```python
from build123d import *

# Parameters (mm, degrees)
BOSS_EXTRUDE1_DEPTH = 14.5
SKETCH3_R           = 4.1
CUT_EXTRUDE1_DEPTH  = 4
BOSS_EXTRUDE2_START = 2
SKETCH5_R           = 14.5
SKETCH5_R_2         = 4.1
BOSS_EXTRUDE2_DEPTH = 2
SKETCH6_R           = 1.55
CUT_EXTRUDE3_DEPTH  = 3
SKETCH7_R           = 10.5
CUT_EXTRUDE4_DEPTH  = 3
FILLET1_R           = 14.5
CUT_EXTRUDE5_DEPTH  = 3
SKETCH9_R           = 1.55
CUT_EXTRUDE6_DEPTH  = 3
SKETCH10_R          = 3
CUT_EXTRUDE7_DEPTH  = 2
SKETCH13_W          = 33
SKETCH13_H          = 3
CUT_EXTRUDE8_DEPTH  = 29


with BuildPart() as part:
    # Sketch2 → Boss-Extrude1 (new, symmetric)
    with BuildSketch(Plane.XY):
        Polygon((-63.7, 18.3), (-4.658041958, 18.3), (10, 3), (43, 3), (43, 0), (0, 0), (-13.7, 14.3), (-63.7, 14.3), align=None)
    extrude(amount=BOSS_EXTRUDE1_DEPTH, both=True)

    # Sketch3 → Cut-Extrude1 (cut)
    with BuildSketch(Plane(origin=(0, 18.3, 0), x_dir=(1, 0, 0), z_dir=(0, 1, 0))):
        with Locations(Location((-49.2, 0, 0), (0, 0, 270))):
            Circle(SKETCH3_R)
    extrude(amount=-CUT_EXTRUDE1_DEPTH, mode=Mode.SUBTRACT)

    # Sketch5 → Boss-Extrude2 (add)
    with BuildSketch(Plane(origin=(0, 18.3, 0), x_dir=(1, 0, 0), z_dir=(0, 1, 0)).offset(BOSS_EXTRUDE2_START)):
        with Locations(Location((-49.2, 0, 0), (0, 0, 270))):
            Circle(SKETCH5_R)
        with Locations(Location((-49.2, 0, 0), (0, 0, 270))):
            Circle(SKETCH5_R_2, mode=Mode.SUBTRACT)
    extrude(amount=-BOSS_EXTRUDE2_DEPTH)

    # Sketch6 → Cut-Extrude3 (cut)
    with BuildSketch(Plane(origin=(0, 3, 0), x_dir=(1, 0, 0), z_dir=(0, 1, 0))):
        with Locations(Location((22.248092992, -5.560176775, 0), (0, 0, 180))):
            Circle(SKETCH6_R)
        with Locations(Location((33.751907008, 5.560176775, 0), (0, 0, 180))):
            Circle(SKETCH6_R)
    extrude(amount=-CUT_EXTRUDE3_DEPTH, mode=Mode.SUBTRACT)

    # Sketch7 → Cut-Extrude4 (cut)
    with BuildSketch(Plane.XZ.offset(-14.3)):
        with Locations((-49.2, 0)):
            Circle(SKETCH7_R)
    extrude(amount=-CUT_EXTRUDE4_DEPTH, mode=Mode.SUBTRACT)

    # Fillet1
    fillet1_edges = [part.edges().sort_by_distance(p)[0] for p in [
        (-63.7, 16.3, -14.5),
        (-63.7, 16.3, 14.5),
    ]]
    fillet(fillet1_edges, radius=FILLET1_R - 0.0001)  # a hair under: the kernel refuses the full size

    # Sketch8 → Cut-Extrude5 (cut)
    with BuildSketch(Plane(origin=(0, 3, 0), x_dir=(1, 0, 0), z_dir=(0, 1, 0))):
        Polygon((16, -3.5), (10, -14.5), (16, -14.5), (43, -14.5), (43, -3.5), align=None)
    extrude(amount=-CUT_EXTRUDE5_DEPTH, mode=Mode.SUBTRACT)

    # Sketch9 → Cut-Extrude6 (cut)
    with BuildSketch(Plane(origin=(0, 3, 0), x_dir=(1, 0, 0), z_dir=(0, 1, 0))):
        with Locations(Location((22.251907008, 5.560176775, 0), (0, 0, 270))):
            Circle(SKETCH9_R)
    extrude(amount=-CUT_EXTRUDE6_DEPTH, mode=Mode.SUBTRACT)

    # Sketch10 → Cut-Extrude7 (cut)
    with BuildSketch(Plane.XZ):
        with Locations((22.251907008, -5.560176775)):
            Circle(SKETCH10_R)
        with Locations((33.751907008, -5.560176775)):
            Circle(SKETCH10_R)
    extrude(amount=-CUT_EXTRUDE7_DEPTH, mode=Mode.SUBTRACT)

    # Sketch13 → Cut-Extrude8 (cut)
    with BuildSketch(Plane(origin=(0, 0, -14.5), x_dir=(-1, 0, 0), z_dir=(0, 0, -1))):
        with Locations((-26.5, 1.5)):
            Rectangle(SKETCH13_W, SKETCH13_H)
    extrude(amount=-CUT_EXTRUDE8_DEPTH, mode=Mode.SUBTRACT)


solid = part.part
```
Input: part model. Units: mm. Frame: model coordinates. A direction names the side the tool comes from. Coordinates: 2 decimals unless noted, no trailing zeros. Loops run counter-clockwise (first coordinate to the right, second up) from the corner with the lowest first, then second, coordinate; pieces in that order, holes last. Notation, with made-up numbers: M 39.5,52 L 78.5,52 A16 cw 78.5,79 Z; hole C 27.25,62.25 d3. An arc over 180 degrees is marked long. One line per item, written item: value.
(1) Reachability of faces 1 (the flat face through (-33, 14.3, 0)), 2 (the flat face through (-52.22, 20.3, 3.02)), 3 (the cylindrical face through (-62.064, 19.314, 6.691)), 4 (the flat face through (-49, 17.3, -5)), 5 (the cylindrical face through (-59.565, 16.328, -10.14)) from +Z, -Z, +X, -X, +Y, -Y: full face, straight path, thin tool, end or side. Return the list, or none.
Filled in:
face 1: +Z, -Z, -X, -Y
face 2: +Z, -Z, +X, -X, +Y
face 3: +Y
face 4: -Y
face 5: -Z, -X, +Y, -Y
(2) Section D-D (x = -37.5). Output: boundary loops of the cut face in (y, z), and give its area (3 significant figures).
Filled in:
outline: M 14.3,-14.5 L 18.3,-14.5 L 18.3,-8.57 L 20.3,-8.57 L 20.3,8.57 L 18.3,8.57 L 18.3,14.5 L 14.3,14.5 Z
area: 150 mm^2
(3) Line query: line 1 along Z through (x, y) = (-49.2, 15.55); line 2 along X through (y, z) = (19, 0); line 3 along Y through (x, z) = (-58.5, 3.75). Output: solid intervals per line, ascending. Write a range as from..to.
Filled in:
line 1: -14.5..-10.5, 10.5..14.5
line 2: -63.7..-53.3, -45.1..-34.7
line 3: 17.3..20.3
(4) Pin query (flat end, axial travel): pin 1 (12 mm diameter, centred on y = 14, z = -10, fed in from +X); pin 2 (1.5 mm diameter, centred on y = 17.5, z = 6, fed in from -X); pin 3 (5 mm diameter, centred on x = -4.5, z = -7.5, fed in from -Y). Return the tip coordinate at first contact, or that it passes through.
Filled in:
pin 1: x = 5.21
pin 2: x = -62.72
pin 3: y = 2.09
(5) Pull-direction query (X, two-part tool) for faces 6 (the flat face through (2.568, 10.757, 0.203)), 7 (the cylindrical face through (-39.2, 15.8, 3.2)), 8 (the flat face through (-11, 12, 14.5)); classes: +X half, -X half, draft (parallel to the pull), parting line (faces both ways), or undercut.
Filled in:
face 6: +X half
face 7: undercut
face 8: draft
